Geometry check sheet. Reference: drawing and pictorial views, mm from the part's lowest x, y, z. A direction names the side the tool comes from. Coordinates: 2 decimals unless noted, no trailing zeros. Loops run counter-clockwise (first coordinate to the right, second up) from the corner with the lowest first, then second, coordinate; pieces in that order, holes last.
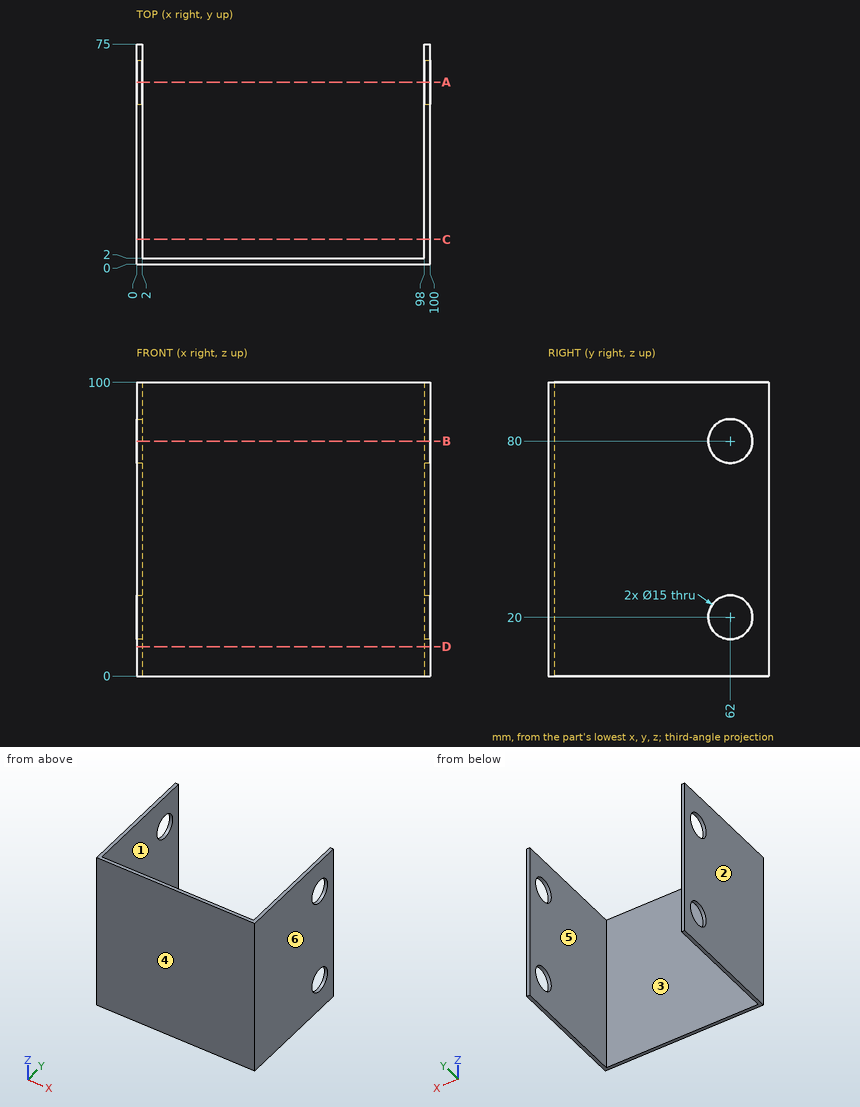
1) Depth check by flat-ended pin: pin 1 (1.5 mm diameter, centred on x = 57.5, z = 48.5, fed in from +Y); pin 2 (13.5 mm diameter, centred on y = 62, z = 80, fed in from +X). Enter the tip coordinate at first touch or a pass-through.
Data:
pin 1: stops at y = 2
pin 2: passes through
2) Section check A-A on y = 62. Record the cut outline in (x, z).
Data:
outline: (0, 0) - (2, 0) - (2, 12.5) - (0, 12.5) - close; (0, 27.5) - (2, 27.5) - (2, 72.5) - (0, 72.5) - close; (0, 87.5) - (2, 87.5) - (2, 100) - (0, 100) - close; (98, 0) - (100, 0) - (100, 12.5) - (98, 12.5) - close; (98, 27.5) - (100, 27.5) - (100, 72.5) - (98, 72.5) - close; (98, 87.5) - (100, 87.5) - (100, 100) - (98, 100) - close
3) Section check C-C on y = 8.5. Record the cut outline in (x, z).
Data:
outline: (0, 0) - (2, 0) - (2, 100) - (0, 100) - close; (98, 0) - (100, 0) - (100, 100) - (98, 100) - close
4) Mould release check, pull along X, two halves, no side actions. Record for the marked faces 1, 2, 3 and 4: +X half, -X half, draft (parallel to the pull), parting line (faces both ways), or undercut.
Data:
face 1: undercut
face 2: -X half
face 3: undercut
face 4: draft
5) Section check B-B on z = 80. Record the cut outline in (x, y), and give its area (3 significant figures).
Data:
outline: (0, 0) - (100, 0) - (100, 54.5) - (98, 54.5) - (98, 2) - (2, 2) - (2, 54.5) - (0, 54.5) - close; (0, 69.5) - (2, 69.5) - (2, 75) - (0, 75) - close; (98, 69.5) - (100, 69.5) - (100, 75) - (98, 75) - close
area: 432 mm2
6) Section check D-D on z = 10. Record the cut outline in (x, y).
Data:
outline: (0, 0) - (100, 0) - (100, 75) - (98, 75) - (98, 2) - (2, 2) - (2, 75) - (0, 75) - close
7) Access from +Z, -Z, +X, -X, +Y, -Y to the whole of each face (thin tool, end or side, straight path). Record for the marked faces 5 and 6.
Data:
face 5: +Z, -Z, +Y
face 6: +Z, -Z, +X, +Y, -Y
8) Material ranges on probe 1 along Z at (x, y) = (99, 62); probe 2 along X at (y, z) = (26, 84.5); probe 3 along Y at (x, z) = (0.45, 80), recorded low to high.
Data:
probe 1: z = 0 to 12.5, 27.5 to 72.5, 87.5 to 100
probe 2: x = 0 to 2, 98 to 100
probe 3: y = 0 to 54.5, 69.5 to 75
